from build123d import *

# Parameters (mm, degrees)
F1_DEPTH = 21
F0_R     = 1
F0_W     = 12.36
F0_H     = 4.61
F2_DEPTH = 2
F3_DEPTH = 6
F4_R     = 2.35
F5_DEPTH = 6.85


with BuildPart() as f1:
    # F0 (on Front) → F1 (new body)
    with BuildSketch(Plane.XZ):
        with BuildLine():
            Line((0, 11.5), (-6.18, 11.5))
            Line((-6.18, 11.5), (-6.18, 5.32))
            ThreePointArc((-6.18, 5.32), (-4.3699199077, 9.6899199077), (0, 11.5))
        make_face()
        with BuildLine():
            ThreePointArc((6.18, 5.32), (0, -0.86), (-6.18, 5.32))
            Line((-6.18, 5.32), (-6.18, -11.5))
            Line((-6.18, -11.5), (6.18, -11.5))
            Line((6.18, -11.5), (6.18, 5.32))
        make_face()
        with BuildLine():
            Line((6.18, 5.32), (6.18, 11.5))
            Line((6.18, 11.5), (0, 11.5))
            ThreePointArc((0, 11.5), (4.3699199077, 9.6899199077), (6.18, 5.32))
        make_face()
        with BuildLine():
            ThreePointArc((0, 11.5), (-4.3699199077, 9.6899199077), (-6.18, 5.32))
            ThreePointArc((-6.18, 5.32), (0, -0.86), (6.18, 5.32))
            ThreePointArc((6.18, 5.32), (4.3699199077, 9.6899199077), (0, 11.5))
        make_face()
    extrude(amount=-F1_DEPTH)

    # F0 (on Front) → F2 (join)
    with BuildSketch(Plane.XZ):
        Polygon((6.18, 16.11), (-6.18, 16.11), (-6.18, 11.5), (0, 11.5), (6.18, 11.5), align=None)
        with Locations((0, 13.805)):
            Circle(F0_R, mode=Mode.SUBTRACT)
        with Locations((0, -13.805)):
            Rectangle(F0_W, F0_H)
        with Locations((0, -13.805)):
            Circle(F0_R, mode=Mode.SUBTRACT)
    extrude(amount=-F2_DEPTH)

    # F0 (on Front) → F3 (join)
    with BuildSketch(Plane.XZ):
        with BuildLine():
            ThreePointArc((0, 11.5), (-4.3699199077, 9.6899199077), (-6.18, 5.32))
            ThreePointArc((-6.18, 5.32), (0, -0.86), (6.18, 5.32))
            ThreePointArc((6.18, 5.32), (4.3699199077, 9.6899199077), (0, 11.5))
        make_face()
    extrude(amount=F3_DEPTH)

    # F4 (on face) → F5 (join)
    with BuildSketch(Plane.XZ.offset(6)):
        with Locations((0, 5.32)):
            Circle(F4_R)
    extrude(amount=F5_DEPTH)


solid = f1.part
Can you work these out from the model? Positions are in its coordinate system, mm. A direction names the side the tool comes from. Coordinates: 2 decimals unless noted, no trailing zeros. Write each loop counter-clockwise with the first axis right and the second up, starting at its lowest first coordinate (ties: lowest second). Pieces come first, ordered by that corner, then holes. Notation, with made-up numbers: M -2.75,-1.75 L 17.25,-1.75 A22 ccw 17.25,14.25 Z; hole C 49,63 d1. An arc over 180 degrees is marked long. Use one line per item in the form item = value.
Q1. We'd pull the mould along Z, two halves only. Please class faces 5 (the flat face through (0, 0, 12)), 6 (the cylindrical face through (-0.22, 0.99, 12.83)), 7 (the cylindrical face through (-0.509, -9.377, 3.026)): +Z half, -Z half, draft (parallel to the pull), parting line (faces both ways), or undercut.
Model answer:
face_5 = draft
face_6 = undercut
face_7 = parting line
Q2. If we section it at B-B (z = -2): Write out the boundary of the cut face in (x, y), then the cut area to 3 significant figures.
Model answer:
outline = M -6.18,0 L 6.18,0 L 6.18,21 L -6.18,21 Z
area = 260 mm^2
Q3. If we section it at C-C (y = 13): Write out the boundary of the cut face in (x, z), then the cut area to 3 significant figures.
Model answer:
outline = M -6.18,-11.5 L 6.18,-11.5 L 6.18,11.5 L -6.18,11.5 Z
area = 284 mm^2
Q4. I need wall thicknesses on line 1 along Z through (x, y) = (0, 0.9) (3 decimals); line 2 along Y through (x, z) = (5, -13); line 3 along Z through (x, y) = (1, 8). Which ranges of each line are inside material? Lowest first, please. Write a range as from..to.
Model answer:
line_1 = -16.11..-14.805, -12.805..12.805, 14.805..16.11
line_2 = 0..2
line_3 = -11.5..11.5
Q5. If we section it at A-A (x = 5.25): Write out the boundary of the cut face in (y, z).
Model answer:
outline = M -6,2.06 L 0,2.06 L 0,-16.11 L 2,-16.11 L 2,-11.5 L 21,-11.5 L 21,11.5 L 2,11.5 L 2,16.11 L 0,16.11 L 0,8.58 L -6,8.58 Z
Q6. For P1, Ø3, axis at x = 0, z = 13.805, coming from the -Y side; P2, Ø4, axis at x = 2, y = -2.5, coming from the +Z side; P3, Ø4, axis at x = 1, y = -8.5, coming from the +Z side; P4, Ø6, axis at y = -2, z = 6, coming from the +X side, each with a flat end and sliding along its axis, tell me the tip position at first contact or that it passes through.
Model answer:
P1 = 0
P2 = 11.5
P3 = 7.67
P4 = 6.18
Q7. If we section it at D-D (x = 1.5): Write out the boundary of the cut face in (y, z).
Model answer:
outline = M -12.85,3.51 L -6,3.51 L -6,-0.68 L 0,-0.68 L 0,-16.11 L 2,-16.11 L 2,-11.5 L 21,-11.5 L 21,11.5 L 2,11.5 L 2,16.11 L 0,16.11 L 0,11.32 L -6,11.32 L -6,7.13 L -12.85,7.13 Z
Q8. For faces 1 (the flat face through (0, 11, -11.5)), 2 (the flat face through (0, 11, 11.5)), 3 (the flat face through (3, -6, 5)), 4 (the flat face through (6.18, 10, 0)), which set-ups out of +Z, -Z, +X, -X, +Y, -Y let a thin tool reach every point of the face, with its end or its side?
Model answer:
face_1 = -Z, +X, -X, +Y
face_2 = +Z, +X, -X, +Y
face_3 = -Y
face_4 = +Z, -Z, +X, +Y, -Y
